from build123d import *

# Parameters (mm, degrees)
F0_R     = 1.575
F0_R_2   = 5.5
F1_DEPTH = 14
F3_R     = 4.25
F4_DEPTH = 200
F5_W     = 5
F5_H     = 23.55
F6_DEPTH = 14
F7_DEPTH = 25


with BuildPart() as f1:
    # F0 (on Top) → F1 (new body)
    with BuildSketch(Plane.XY):
        with BuildLine():
            Line((-25, -15), (0, -15))
            Line((0, -15), (25, -15))
            Line((25, -15), (25, 0))
            Line((25, 0), (25, 124.1133357109))
            ThreePointArc((25, 124.1133357109), (22.2130258043, 124.0468770319), (20.8, 126.45))
            Line((20.8, 126.45), (-20.8, 126.45))
            ThreePointArc((-20.8, 126.45), (-22.2130258043, 124.0468770319), (-25, 124.1133357109))
            Line((-25, 124.1133357109), (-25, 0))
            Line((-25, 0), (-25, -15))
        make_face()
        with Locations((-5.657, -5.656855)):
            Circle(F0_R, mode=Mode.SUBTRACT)
        with Locations((-5.657, 5.656855)):
            Circle(F0_R, mode=Mode.SUBTRACT)
        with Locations((5.657, -5.656855)):
            Circle(F0_R, mode=Mode.SUBTRACT)
        Circle(F0_R_2, mode=Mode.SUBTRACT)
        with Locations((5.657, 5.656855)):
            Circle(F0_R, mode=Mode.SUBTRACT)
        with BuildLine():
            Line((-20.8, 126.45), (20.8, 126.45))
            ThreePointArc((20.8, 126.45), (21.6054563517, 128.3945436483), (23.55, 129.2))
            Line((23.55, 129.2), (23.55, 145))
            Line((23.55, 145), (10.3561575886, 145))
            ThreePointArc((10.3561575886, 145), (0, 138.5), (-10.3561575886, 145))
            Line((-10.3561575886, 145), (-23.55, 145))
            Line((-23.55, 145), (-23.55, 129.2))
            ThreePointArc((-23.55, 129.2), (-21.6054563517, 128.3945436483), (-20.8, 126.45))
        make_face()
        with BuildLine():
            Line((-25, 145), (-25, 128.7866642891))
            ThreePointArc((-25, 128.7866642891), (-24.3038810267, 129.0946480669), (-23.55, 129.2))
            Line((-23.55, 129.2), (-23.55, 145))
            Line((-23.55, 145), (-25, 145))
        make_face()
        with BuildLine():
            ThreePointArc((23.55, 129.2), (24.3038810267, 129.0946480669), (25, 128.7866642891))
            Line((25, 128.7866642891), (25, 145))
            Line((25, 145), (23.55, 145))
            Line((23.55, 145), (23.55, 129.2))
        make_face()
    extrude(amount=F1_DEPTH)

    # F3 (on offset) → F4 (cut)
    with BuildSketch(Plane.XZ.offset(15)):
        with Locations((-14, 7)):
            Circle(F3_R)
        with Locations((14, 7)):
            Circle(F3_R)
    extrude(amount=-F4_DEPTH, mode=Mode.SUBTRACT)

    # F5 (on Top) → F6 (join)
    with BuildSketch(Plane.XY):
        with Locations((27.5, 133.225)):
            Rectangle(F5_W, F5_H)
        with Locations((-27.5, 133.225)):
            Rectangle(F5_W, F5_H)
    extrude(amount=F6_DEPTH)

    # F0 (on Top) → F7 (cut)
    with BuildSketch(Plane.XY):
        with BuildLine():
            ThreePointArc((20.8, 126.45), (22.2130258043, 124.0468770319), (25, 124.1133357109))
            Line((25, 124.1133357109), (25, 128.7866642891))
            ThreePointArc((25, 128.7866642891), (24.3038810267, 129.0946480669), (23.55, 129.2))
            Line((23.55, 129.2), (23.55, 126.45))
            Line((23.55, 126.45), (20.8, 126.45))
        make_face()
        with BuildLine():
            Line((25, 128.7866642891), (25, 124.1133357109))
            ThreePointArc((25, 124.1133357109), (25.9531229681, 125.1130258043), (26.3, 126.45))
            ThreePointArc((26.3, 126.45), (25.9531229681, 127.7869741957), (25, 128.7866642891))
        make_face()
        with BuildLine():
            ThreePointArc((23.55, 129.2), (21.6054563517, 128.3945436483), (20.8, 126.45))
            Line((20.8, 126.45), (23.55, 126.45))
            Line((23.55, 126.45), (23.55, 129.2))
        make_face()
        with BuildLine():
            ThreePointArc((-25, 128.7866642891), (-26.3, 126.45), (-25, 124.1133357109))
            Line((-25, 124.1133357109), (-25, 128.7866642891))
        make_face()
        with BuildLine():
            Line((-25, 128.7866642891), (-25, 124.1133357109))
            ThreePointArc((-25, 124.1133357109), (-22.2130258043, 124.0468770319), (-20.8, 126.45))
            Line((-20.8, 126.45), (-23.55, 126.45))
            Line((-23.55, 126.45), (-23.55, 129.2))
            ThreePointArc((-23.55, 129.2), (-24.3038810267, 129.0946480669), (-25, 128.7866642891))
        make_face()
        with BuildLine():
            Line((-23.55, 126.45), (-20.8, 126.45))
            ThreePointArc((-20.8, 126.45), (-21.6054563517, 128.3945436483), (-23.55, 129.2))
            Line((-23.55, 129.2), (-23.55, 126.45))
        make_face()
    extrude(amount=F7_DEPTH, mode=Mode.SUBTRACT)


solid = f1.part
The model under review builds one solid part; all positions refer to its coordinate system, in mm. A direction names the side the tool comes from. Coordinates: 2 decimals unless noted, no trailing zeros. Write each loop counter-clockwise with the first axis right and the second up, starting at its lowest first coordinate (ties: lowest second). Pieces come first, ordered by that corner, then holes. Notation, with made-up numbers: M 80.25,-5.5 L 132.25,-5.5 A16 cw 132.25,13.5 Z; hole C 13.5,72.25 d3. An arc over 180 degrees is marked long. Put each result on its own line as item: value.
1) Clearance check with flat-ended pins moving along their axes: pin 1 Ø1.5 at (x, z) = (-28.5, 5.5) entering from -Y; pin 2 Ø4 at (y, z) = (28, 10) entering from +X; pin 3 Ø5 at (y, z) = (101.5, 7) entering from -X; pin 4 Ø7.5 at (x, z) = (-14, 7) entering from +Y. State where each tip first meets the part, or that it passes through.
Computed:
pin 1: stops at y = 121.45
pin 2: stops at x = 25
pin 3: stops at x = -25
pin 4: passes through
2) Add section D-D on z = 7. State how many separate pieces and enclosed holes the cut face has, then the cut area to 3 significant figures.
Computed:
separate pieces: 3
enclosed holes: 7
area: 5,250 mm2
3) For faces 4 (the flat face through (25, 52, 7)), 5 (the flat face through (-28, 121.45, 7)), 6 (the flat face through (0, 66, 14)), list the 3-axis set-ups (+Z, -Z, +X, -X, +Y, -Y) from which the entire face can be reached by the end or side of a thin tool; tool diameter is ignored.
Computed:
face 4: +Z, -Z, +X, -Y
face 5: +Z, -Z, -X, -Y
face 6: +Z, +X, -X, +Y, -Y
4) Draft analysis for pull direction X (two halves, no side actions). For faces 1 (the flat face through (27, 121.45, 7)), 2 (the flat face through (-30, 133, 7)), 3 (the cylindrical face through (-6, 4.12, 6.9)), state which applies: released by +X, released by -X, zero draft, split by the parting line, or undercut.
Computed:
face 1: zero draft
face 2: released by -X
face 3: undercut
5) Wall thickness on probe 1 along X at (y, z) = (47, 7); probe 2 along X at (y, z) = (95, 5.75); probe 3 along Y at (x, z) = (-5, 1.25): over which ranges is each line inside the solid? List them lowest first. Write a range as [from, to].
Computed:
probe 1: x = [-25, -18.25], [-9.75, 9.75], [18.25, 25]
probe 2: x = [-25, -18.06], [-9.94, 9.94], [18.06, 25]
probe 3: y = [-15, -7.09], [-4.23, -2.29], [2.29, 4.23], [7.09, 139.64]
6) Add section C-C on y = 35. Give the boundary of the cut face in (x, z).
Computed:
outline: M -25,0 L 25,0 L 25,14 L -25,14 Z; hole C -14,7 d8.5; hole C 14,7 d8.5
7) Add section B-B on x = 0. Give the boundary of the cut face in (y, z), then the cut area to 4 significant figures.
Computed:
outline: M -15,0 L -5.5,0 L -5.5,14 L -15,14 Z; M 5.5,0 L 138.5,0 L 138.5,14 L 5.5,14 Z
area: 1,995 mm2
8) Add section A-A on y = 0. Give the boundary of the cut face in (x, z), then the cut area to 3 significant figures.
Computed:
outline: M -25,0 L -5.5,0 L -5.5,14 L -25,14 Z; M 5.5,0 L 25,0 L 25,14 L 5.5,14 Z; hole C -14,7 d8.5; hole C 14,7 d8.5
area: 433 mm2
